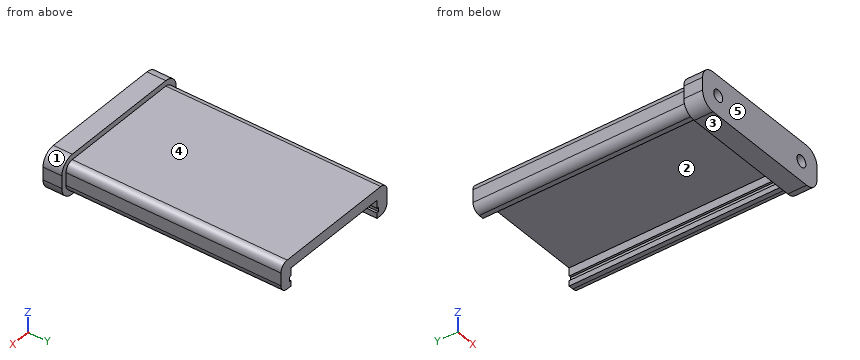
```python
from build123d import *

# Parameters (mm, degrees)
SKETCH2_W               = 88.9
SKETCH2_H               = 152.4
BOSS_EXTRUDE1_DEPTH     = 5.9944
SKETCH4_R               = 2.7305
CUT_EXTRUDE2_DEPTH      = 1
CUT_EXTRUDE2_DEPTH_BACK = 6.9944
BOSS_EXTRUDE2_DEPTH     = 101.6
FILLET1_R               = 3.81
SKETCH7_W               = 2.54
SKETCH7_H               = 152.4
CUT_EXTRUDE3_DEPTH      = 102.6
CUT_EXTRUDE3_DEPTH_BACK = 6.9944
SKETCH11_W              = 86.36
SKETCH11_H              = 152.4
CUT_EXTRUDE4_DEPTH      = 6.35
BOSS_EXTRUDE3_DEPTH     = 8.89
SKETCH13_R              = 2.7305
CUT_EXTRUDE5_DEPTH      = 6.35


with BuildPart() as part:
    # Sketch2 → Boss-Extrude1 (new body)
    with BuildSketch(Plane(origin=(0, 0, 0), x_dir=(1, 0, 0), z_dir=(0, 1, 0))):
        with Locations((44.45, 76.2)):
            Rectangle(SKETCH2_W, SKETCH2_H)
    extrude(amount=BOSS_EXTRUDE1_DEPTH)

    # Sketch4 → Cut-Extrude2 (cut, two sides)
    with BuildSketch(Plane(origin=(0, 5.9944, 0), x_dir=(1, 0, 0), z_dir=(0, 1, 0))) as cut_extrude2_sk:
        with Locations((45.72, 109.871331367)):
            Circle(SKETCH4_R)
        with Locations((45.72, 33.671331367)):
            Circle(SKETCH4_R)
    extrude(amount=CUT_EXTRUDE2_DEPTH, mode=Mode.SUBTRACT)
    extrude(cut_extrude2_sk.sketch, amount=-CUT_EXTRUDE2_DEPTH_BACK, mode=Mode.SUBTRACT)

    # Sketch5 → Boss-Extrude2 (add)
    with BuildSketch(Plane(origin=(0, 5.9944, 0), x_dir=(1, 0, 0), z_dir=(0, 1, 0))):
        Polygon((18.161, 16.129), (12.065, 16.129), (12.065, 2.54), (76.835, 2.54), (76.835, 16.129), (70.739, 16.129), (70.739, 13.589), (71.755, 13.589), (71.755, 11.43), (70.739, 11.43), (70.739, 7.62), (18.161, 7.62), (18.161, 11.43), (17.145, 11.43), (17.145, 13.589), (18.161, 13.589), align=None)
    extrude(amount=BOSS_EXTRUDE2_DEPTH)

    # Fillet1
    fillet1_edges = [part.edges().sort_by_distance(p)[0] for p in [
        (12.065, 56.7944, -16.129),
        (12.065, 56.7944, -2.54),
        (76.835, 56.7944, -2.54),
        (76.835, 56.7944, -16.129),
    ]]
    fillet(fillet1_edges, radius=FILLET1_R)

    # Sketch7 → Cut-Extrude3 (cut, two sides)
    with BuildSketch(Plane(origin=(0, 5.9944, 0), x_dir=(1, 0, 0), z_dir=(0, 1, 0))) as cut_extrude3_sk:
        with Locations((1.27, 76.2)):
            Rectangle(SKETCH7_W, SKETCH7_H)
    extrude(amount=CUT_EXTRUDE3_DEPTH, mode=Mode.SUBTRACT)
    extrude(cut_extrude3_sk.sketch, amount=-CUT_EXTRUDE3_DEPTH_BACK, mode=Mode.SUBTRACT)

    # Sketch11 → Cut-Extrude4 (cut)
    with BuildSketch(Plane.XZ):
        with Locations((45.72, -76.2)):
            Rectangle(SKETCH11_W, SKETCH11_H)
    extrude(amount=-CUT_EXTRUDE4_DEPTH, mode=Mode.SUBTRACT)

    # Sketch12 → Boss-Extrude3 (add)
    with BuildSketch(Plane.XZ.offset(-6.35)):
        with BuildLine():
            Line((9.525, -6.35), (9.525, -12.319))
            ThreePointArc((9.525, -12.319), (11.384871939, -16.809128061), (15.875, -18.669))
            Line((15.875, -18.669), (18.161, -18.669))
            Line((18.161, -18.669), (70.739, -18.669))
            Line((70.739, -18.669), (73.025, -18.669))
            ThreePointArc((73.025, -18.669), (77.515128061, -16.809128061), (79.375, -12.319))
            Line((79.375, -12.319), (79.375, -6.35))
            ThreePointArc((79.375, -6.35), (77.515128061, -1.859871939), (73.025, 0))
            Line((73.025, 0), (15.875, 0))
            ThreePointArc((15.875, 0), (11.384871939, -1.859871939), (9.525, -6.35))
        make_face()
        with BuildLine():
            Line((18.161, -16.129), (70.739, -16.129))
            Line((70.739, -16.129), (73.025, -16.129))
            ThreePointArc((73.025, -16.129), (75.719076836, -15.013076836), (76.835, -12.319))
            Line((76.835, -12.319), (76.835, -6.35))
            ThreePointArc((76.835, -6.35), (75.719076836, -3.655923164), (73.025, -2.54))
            Line((73.025, -2.54), (15.875, -2.54))
            ThreePointArc((15.875, -2.54), (13.180923164, -3.655923164), (12.065, -6.35))
            Line((12.065, -6.35), (12.065, -12.319))
            ThreePointArc((12.065, -12.319), (13.180923164, -15.013076836), (15.875, -16.129))
            Line((15.875, -16.129), (18.161, -16.129))
        make_face(mode=Mode.SUBTRACT)
        with BuildLine():
            Line((70.739, -11.43), (71.755, -11.43))
            Line((71.755, -11.43), (71.755, -13.589))
            Line((71.755, -13.589), (70.739, -13.589))
            Line((70.739, -13.589), (70.739, -16.129))
            Line((70.739, -16.129), (73.025, -16.129))
            ThreePointArc((73.025, -16.129), (75.719076836, -15.013076836), (76.835, -12.319))
            Line((76.835, -12.319), (76.835, -6.35))
            ThreePointArc((76.835, -6.35), (75.719076836, -3.655923164), (73.025, -2.54))
            Line((73.025, -2.54), (15.875, -2.54))
            ThreePointArc((15.875, -2.54), (13.180923164, -3.655923164), (12.065, -6.35))
            Line((12.065, -6.35), (12.065, -12.319))
            ThreePointArc((12.065, -12.319), (13.180923164, -15.013076836), (15.875, -16.129))
            Line((15.875, -16.129), (18.161, -16.129))
            Line((18.161, -16.129), (18.161, -13.589))
            Line((18.161, -13.589), (17.145, -13.589))
            Line((17.145, -13.589), (17.145, -11.43))
            Line((17.145, -11.43), (18.161, -11.43))
            Line((18.161, -11.43), (18.161, -7.62))
            Line((18.161, -7.62), (70.739, -7.62))
            Line((70.739, -7.62), (70.739, -11.43))
        make_face()
        Polygon((18.161, -16.129), (70.739, -16.129), (70.739, -13.589), (71.755, -13.589), (71.755, -11.43), (70.739, -11.43), (70.739, -7.62), (18.161, -7.62), (18.161, -11.43), (17.145, -11.43), (17.145, -13.589), (18.161, -13.589), align=None)
    extrude(amount=BOSS_EXTRUDE3_DEPTH)

    # Sketch13 → Cut-Extrude5 (cut)
    with BuildSketch(Plane.XZ.offset(2.54)):
        with Locations((19.05, -9.3345)):
            Circle(SKETCH13_R)
        with Locations((69.85, -9.3345)):
            Circle(SKETCH13_R)
    extrude(amount=-CUT_EXTRUDE5_DEPTH, mode=Mode.SUBTRACT)


solid = part.part
```
For this review, take the finished solid that the model builds, in its own axes (mm). Face numbers are marked on the shaded views. A direction names the side the tool comes from. Round coordinates to 2 decimals unless told otherwise and drop trailing zeros. Write each loop counter-clockwise with the first axis right and the second up, starting at its lowest first coordinate (ties: lowest second). Pieces come first, ordered by that corner, then holes. Notation, with made-up numbers: M 20,-27 L 66,-27 A16 cw 66,0 Z; hole C -14.5,21 d9. An arc over 180 degrees is marked long. One line per item, written item: value. Start each with the question number.
(1) We need section B-B (y = 48). Give the boundary of the cut face in (x, z) (3 decimals).
(2) We need section A-A (x = 39.5). Give the boundary of the cut face in (y, z), and give its area (3 significant figures).
(3) Wall thickness on line 1 (Z direction, x = 19, y = 0); line 2 (X direction, y = 84.5, z = -9.5) (3 decimals); line 3 (X direction, y = 62.5, z = -12.25) (3 decimals): over which ranges is each line inside the solid? List them lowest first.
(4) Machinability: for the marked faces 4 and 5, which of the approach directions +Z, -Z, +X, -X, +Y, -Y give a long, thin tool a straight path to every point of the face, cutting with its end or side? Answer none if there is none.
(5) The part is to be moulded in two halves that separate along X. For the marked faces 1, 2 and 3, say which applies: released by +X, released by -X, zero draft, split by the parting line, or undercut.
(6) Insertion check: pin 1 (0.6 mm diameter, centred on y = 72.5, z = -13, fed in from -X); pin 2 (2 mm diameter, centred on x = 31, z = -16.5, fed in from +Y); pin 3 (5 mm diameter, centred on y = 84, z = -7.5, fed in from +X) (3 decimals). Each pin has a flat end and moves straight along its axis. Give the tip position at first contact, or say it passes through.
Result:
1. outline: M 12.065,-12.319 A3.81 ccw 15.875,-16.129 L 18.161,-16.129 L 18.161,-13.589 L 17.145,-13.589 L 17.145,-11.43 L 18.161,-11.43 L 18.161,-7.62 L 70.739,-7.62 L 70.739,-11.43 L 71.755,-11.43 L 71.755,-13.589 L 70.739,-13.589 L 70.739,-16.129 L 73.025,-16.129 A3.81 ccw 76.835,-12.319 L 76.835,-6.35 A3.81 ccw 73.025,-2.54 L 15.875,-2.54 A3.81 ccw 12.065,-6.35 Z
2. outline: M -2.54,-18.67 L 6.35,-18.67 L 6.35,-7.62 L 107.59,-7.62 L 107.59,-2.54 L 6.35,-2.54 L 6.35,0 L -2.54,0 Z
2. area: 680 mm²
3. line 1: -18.67 to -12.06, -6.6 to 0
3. line 2: 12.065 to 18.161, 70.739 to 76.835
3. line 3: 12.065 to 17.145, 71.755 to 76.835
4. face 4: +Z, +X, -X, +Y
4. face 5: +Z, -Z, +X, -X, -Y
5. face 1: released by +X
5. face 2: undercut
5. face 3: zero draft
6. pin 1: x = 12.08
6. pin 2: y = 6.35
6. pin 3: x = 76.835
